Geometry check sheet. Reference: the model listing, model coordinates, mm. A direction names the side the tool comes from. Give positions to 0.01 mm unless a question says otherwise; leave off trailing zeros. Write each loop counter-clockwise with the first axis right and the second up, starting at its lowest first coordinate (ties: lowest second). Pieces come first, ordered by that corner, then holes. Notation, with made-up numbers: (-37.75, 84.25) - (19.25, 84.25) arc R20 cw to (19.25, 102.25) - close; hole circle Ø8 at (-5.5, 52.25). An arc over 180 degrees is marked (long way). One line per question, with ' | ' between items. Start each with the question number.
Q1. Section check B-B on y = -17. Record the boundary of the cut face in (x, z).
Q2. Set-up check for faces 5 (the face through (15.8, -24.546, 1.5)), 6 (the face through (21, -2.396, 23)), 7 (the face through (25.96, -20.11, 44.75)), 8 (the face through (15.83, -20.11, 1.25)): record each of +Z, -Z, +X, -X, +Y, -Y from which the full face is reachable in a straight line by a thin tool's end or side.
Q3. Section check D-D on z = 24. Record the boundary of the cut face in (x, y), and give its area (3 significant figures).
Q4. Thickness scan on L1, parallel to X at y = -29.05, z = -0.9; L2, parallel to Z at x = 14, y = -14; L3, parallel to X at y = -19, z = 3.5. Record the ranges inside material, lowest first. Write a range as [from, to].
Q5. Gauge pin test, flat ends, axial feed: P1, Ø3.5, axis at x = 38, y = -13.5, coming from the -Z side; P2, Ø4, axis at y = -9.5, z = 16.5, coming from the +X side; P3, Ø0.9, axis at x = 16, z = 45.5, coming from the -Y side. Record the tip position at first contact, or that the pin passes through.
Q6. Section check C-C on x = 25. Record the boundary of the cut face in (y, z).
Q7. Section check A-A on z = -0.9. Record the boundary of the cut face in (x, y), and give its area (3 significant figures).
Q8. Release check for a two-part mould opening along Z. For faces 1 (the face through (9.397, -17, 23)), 2 (the face through (17, -1.396, 23)), 3 (the face through (21, -17, 43.5)), 4 (the face through (21, -12, 46.5)) record: +Z half, -Z half, draft (parallel to the pull), parting line (faces both ways), or undercut.
```python
from build123d import *

# Parameters (mm, degrees)
BOSS_EXTRUDE1_DEPTH  = 3
SKETCH2_W            = 27
SKETCH2_H            = 3
BOSS_EXTRUDE2_DEPTH  = 5
SKETCH3_R            = 2.15
CUT_EXTRUDE1_DEPTH   = 15
SKETCH5_R            = 3
CUT_EXTRUDE3_DEPTH   = 3
SKETCH7_W            = 2
SKETCH7_H            = 29.15
BOSS_EXTRUDE6_DEPTH  = 43.5
SKETCH8_W            = 3
SKETCH8_H            = 29.15
BOSS_EXTRUDE7_DEPTH  = 25
SKETCH9_W            = 27
SKETCH9_H            = 3
BOSS_EXTRUDE8_DEPTH  = 5
SKETCH10_R           = 2.15
CUT_EXTRUDE4_DEPTH   = 15
SKETCH11_W           = 40.5
SKETCH11_H           = 1
BOSS_EXTRUDE9_DEPTH  = 23
SKETCH12_W           = 3
SKETCH12_H           = 29.15
BOSS_EXTRUDE10_DEPTH = 7


with BuildPart() as part:
    # Sketch1 → Boss-Extrude1 (new body)
    with BuildSketch(Plane.XY):
        Polygon((7.396868841, -30.545988075), (34.396868841, -30.545988075), (34.396868841, -3.045988075), (34.396868841, -1.395988075), (7.396868841, -1.395988075), (7.396868841, -3.045988075), align=None)
    extrude(amount=BOSS_EXTRUDE1_DEPTH)

    # Sketch2 → Boss-Extrude2 (add)
    with BuildSketch(Plane(origin=(0, 0, 0), x_dir=(-1, 0, 0), z_dir=(0, 0, -1))):
        with Locations((-20.896868841, -29.045988075)):
            Rectangle(SKETCH2_W, SKETCH2_H)
    extrude(amount=BOSS_EXTRUDE2_DEPTH)

    # Sketch3 → Cut-Extrude1 (cut)
    with BuildSketch(Plane.XZ.offset(30.545988075)):
        with Locations(Location((15.796868841, -0.9, 0), (0, 0, 270))):
            Circle(SKETCH3_R)
        with Locations(Location((25.996868841, -0.9, 0), (0, 0, 270))):
            Circle(SKETCH3_R)
    extrude(amount=-CUT_EXTRUDE1_DEPTH, mode=Mode.SUBTRACT)

    # Sketch5 → Cut-Extrude3 (cut)
    with BuildSketch(Plane(origin=(0, -27.545988075, 0), x_dir=(1, 0, 0), z_dir=(0, 1, 0))):
        with Locations((15.796868841, 0.9)):
            Circle(SKETCH5_R)
        with Locations((25.996868841, 0.9)):
            Circle(SKETCH5_R)
    cut_extrude3 = extrude(amount=CUT_EXTRUDE3_DEPTH, mode=Mode.SUBTRACT)

    # Sketch7 → Boss-Extrude6 (add)
    with BuildSketch(Plane.XY.offset(3)):
        with Locations((8.396868841, -15.970988075)):
            Rectangle(SKETCH7_W, SKETCH7_H)
    boss_extrude6 = extrude(amount=BOSS_EXTRUDE6_DEPTH)

    # Sketch8 → Boss-Extrude7 (add)
    with BuildSketch(Plane(origin=(9.396868841, 0, 0), x_dir=(0, 0, -1), z_dir=(1, 0, 0))):
        with Locations((-45, -15.970988075)):
            Rectangle(SKETCH8_W, SKETCH8_H)
    extrude(amount=BOSS_EXTRUDE7_DEPTH)

    # Sketch9 → Boss-Extrude8 (add)
    with BuildSketch(Plane.XY.offset(46.5)):
        with Locations((20.896868841, -29.045988075)):
            Rectangle(SKETCH9_W, SKETCH9_H)
    extrude(amount=BOSS_EXTRUDE8_DEPTH)

    # Sketch10 → Cut-Extrude4 (cut)
    with BuildSketch(Plane.XZ.offset(30.545988075)):
        with Locations(Location((25.996868841, 46.9, 0), (0, 0, 270))):
            Circle(SKETCH10_R)
        with Locations(Location((15.796868841, 46.9, 0), (0, 0, 270))):
            Circle(SKETCH10_R)
    extrude(amount=-CUT_EXTRUDE4_DEPTH, mode=Mode.SUBTRACT)

    # Mirror1: Cut-Extrude3 across plane
    add(cut_extrude3.mirror(Plane(origin=(0, 0, 23.25), x_dir=(1, 0, 0), z_dir=(0, 0, -1))), mode=Mode.SUBTRACT)

    # Mirror2: Boss-Extrude6 across plane
    add(boss_extrude6.mirror(Plane.ZY.offset(-20.896868841)))

    # Sketch11 → Boss-Extrude9 (add)
    with BuildSketch(Plane.ZY.offset(-32.396868841)):
        with Locations((23.25, -1.895988075)):
            Rectangle(SKETCH11_W, SKETCH11_H)
    extrude(amount=BOSS_EXTRUDE9_DEPTH)

    # Sketch12 → Boss-Extrude10 (add)
    with BuildSketch(Plane(origin=(34.396868841, 0, 0), x_dir=(0, 0, -1), z_dir=(1, 0, 0))):
        with Locations((-26.5, -15.970988075)):
            Rectangle(SKETCH12_W, SKETCH12_H)
    boss_extrude10 = extrude(amount=BOSS_EXTRUDE10_DEPTH)

    # Mirror3: Boss-Extrude10 across plane
    add(boss_extrude10.mirror(Plane.ZY.offset(-20.896868841)))


solid = part.part
```
Working result:
1) outline: (0.4, 25) - (7.4, 25) - (7.4, 0) - (13.84, 0) arc R2.15 cw to (17.75, 0) - (24.04, 0) arc R2.15 cw to (27.95, 0) - (34.4, 0) - (34.4, 25) - (41.4, 25) - (41.4, 28) - (34.4, 28) - (34.4, 46.5) - (28.11, 46.5) arc R2.15 cw to (23.88, 46.5) - (17.91, 46.5) arc R2.15 cw to (13.68, 46.5) - (7.4, 46.5) - (7.4, 28) - (0.4, 28) - close; hole (9.4, 3) - (32.4, 3) - (32.4, 43.5) - (9.4, 43.5) - close
2) face 5: -Z | face 6: -Y | face 7: +Z, -Y | face 8: -Z, -Y
3) outline: (7.4, -30.55) - (9.4, -30.55) - (9.4, -2.4) - (32.4, -2.4) - (32.4, -30.55) - (34.4, -30.55) - (34.4, -1.4) - (7.4, -1.4) - close | area: 140 mm2
4) L1: x = [7.4, 13.65], [17.95, 23.85], [28.15, 34.4] | L2: z = [0, 3], [43.5, 46.5] | L3: x = [7.4, 9.4], [32.4, 34.4]
5) P1: stops at z = 25 | P2: stops at x = 34.4 | P3: stops at y = -15.55
6) outline: (-30.55, -5) - (-27.55, -5) - (-27.55, -2.8) - (-30.55, -2.8) - close; (-30.55, 1) - (-27.55, 1) - (-27.55, 1.93) - (-24.55, 1.93) - (-24.55, 1) - (-15.55, 1) - (-15.55, 0) - (-1.4, 0) - (-1.4, 46.5) - (-15.55, 46.5) - (-15.55, 45) - (-24.55, 45) - (-24.55, 44.57) - (-27.55, 44.57) - (-27.55, 45) - (-30.55, 45) - (-30.55, 43.5) - (-2.4, 43.5) - (-2.4, 3) - (-30.55, 3) - close; (-30.55, 48.8) - (-27.55, 48.8) - (-27.55, 51.5) - (-30.55, 51.5) - close
7) outline: (7.4, -30.55) - (13.65, -30.55) - (13.65, -27.55) - (7.4, -27.55) - close; (17.95, -30.55) - (23.85, -30.55) - (23.85, -27.55) - (17.95, -27.55) - close; (28.15, -30.55) - (34.4, -30.55) - (34.4, -27.55) - (28.15, -27.55) - close | area: 55.2 mm2
8) face 1: undercut | face 2: draft | face 3: undercut | face 4: +Z half
